Geometry check sheet. Reference: the model listing, model coordinates, mm. Coordinates: 2 decimals unless noted, no trailing zeros. Write each loop counter-clockwise with the first axis right and the second up, starting at its lowest first coordinate (ties: lowest second). Pieces come first, ordered by that corner, then holes. Notation, with made-up numbers: (82.25, 62) -> (114.25, 62) arc R10 ccw to (114.25, 69) -> close; hole circle Ø10 at (49.25, -3). An arc over 180 degrees is marked (long way). Answer in a Markdown table with one row per item. Add a question column.
1. Cross-section at C-C on x = 0. Give the number of separate pieces and of enclosed holes in the cut face, and give its area (3 significant figures).
2. Scan lines: L1, parallel to Z at x = 26, y = 0.25; L2, parallel to X at y = 0.75, z = -26; L3, parallel to Z at x = 0, y = 0.7. Record each from-to range of solid material in increasing order. Write a range as from..to.
3. Cross-section at A-A on x = 26. Record the cut outline in (y, z), and give its area (3 significant figures).
4. Cross-section at B-B on z = -26. Record the cut outline in (x, y).
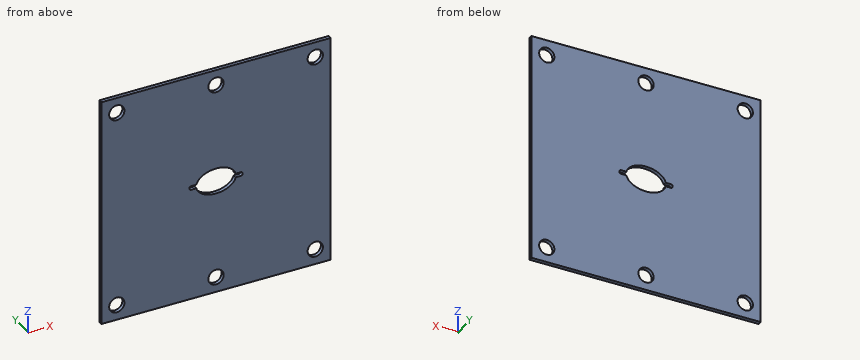
```python
from build123d import *

# Parameters (mm, degrees)
SKETCH1_W                    = 60
SKETCH1_H                    = 60
BOSS_EXTRUDE1_DEPTH          = 1
F_4_0_4_DIAMETER_HOLE1_D     = 4
F_4_0_4_DIAMETER_HOLE1_DEPTH = 1
SKETCH3_R                    = 0.5
CUT_EXTRUDE1_DEPTH           = 5
SKETCH9_W                    = 13
SKETCH9_H                    = 1
CUT_EXTRUDE7_DEPTH           = 5
SKETCH10_RX                  = 5.193553557
SKETCH10_RY                  = 3.369235694
CUT_EXTRUDE8_DEPTH           = 5


with BuildPart() as part:
    # Sketch1 → Boss-Extrude1 (new body)
    with BuildSketch(Plane(origin=(0, 0, 0), x_dir=(1, 0, 0), z_dir=(0, 1, 0))):
        Rectangle(SKETCH1_W, SKETCH1_H)
    extrude(amount=BOSS_EXTRUDE1_DEPTH)

    # Ø4.0 (4) Diameter Hole1
    with Locations(Plane(origin=(0, 1, 0), x_dir=(1, 0, 0), z_dir=(0, 1, 0))):
        with Locations((26, 26), (0, 26), (-26, 26), (0, -26), (26, -26), (-26, -26)):
            Hole(F_4_0_4_DIAMETER_HOLE1_D / 2, depth=F_4_0_4_DIAMETER_HOLE1_DEPTH)

    # Sketch3 → Cut-Extrude1 (cut)
    with BuildSketch(Plane(origin=(0, 1, 0), x_dir=(1, 0, 0), z_dir=(0, 1, 0))):
        with Locations((6.5, 0)):
            Circle(SKETCH3_R)
        with Locations((-6.5, 0)):
            Circle(SKETCH3_R)
    extrude(amount=-CUT_EXTRUDE1_DEPTH, mode=Mode.SUBTRACT)

    # Sketch9 → Cut-Extrude7 (cut)
    with BuildSketch(Plane(origin=(0, 1, 0), x_dir=(1, 0, 0), z_dir=(0, 1, 0))):
        Rectangle(SKETCH9_W, SKETCH9_H)
    extrude(amount=-CUT_EXTRUDE7_DEPTH, mode=Mode.SUBTRACT)

    # Sketch10 → Cut-Extrude8 (cut)
    with BuildSketch(Plane(origin=(0, 1, 0), x_dir=(1, 0, 0), z_dir=(0, 1, 0))):
        with Locations(Location((0, 0), (0, 0, 180))):
            Ellipse(SKETCH10_RX, SKETCH10_RY)
    extrude(amount=-CUT_EXTRUDE8_DEPTH, mode=Mode.SUBTRACT)


solid = part.part
```
Results found:
| question | item | result |
|---|---|---|
| 1 | separate pieces | 4 |
| 1 | enclosed holes | 0 |
| 1 | area | 45.3 mm^2 |
| 2 | L1 | z = -30..-28, -24..24, 28..30 |
| 2 | L2 | x = -30..-28, -24..-2, 2..24, 28..30 |
| 2 | L3 | z = -30..-28, -24..-3.37, 3.37..24, 28..30 |
| 3 | outline | (0, -30) -> (1, -30) -> (1, -28) -> (0, -28) -> close; (0, -24) -> (1, -24) -> (1, 24) -> (0, 24) -> close; (0, 28) -> (1, 28) -> (1, 30) -> (0, 30) -> close |
| 3 | area | 52.0 mm^2 |
| 4 | outline | (-30, 0) -> (-28, 0) -> (-28, 1) -> (-30, 1) -> close; (-24, 0) -> (-2, 0) -> (-2, 1) -> (-24, 1) -> close; (2, 0) -> (24, 0) -> (24, 1) -> (2, 1) -> close; (28, 0) -> (30, 0) -> (30, 1) -> (28, 1) -> close |
